Geometry: final body of the model. Coordinates: model frame, mm. A direction names the side the tool comes from. Give positions to 0.01 mm unless a question says otherwise; leave off trailing zeros. Order: outer loops, then holes, each group sorted by start corner. A loop starts at its lowest first (then second) coordinate and runs counter-clockwise, first axis right, second up. Notation, with made-up numbers: (20, 83.5) - (79, 83.5) arc R29 ccw to (79, 106.5) - close; hole circle Ø6 at (87.25, 8.25). An arc over 180 degrees is marked (long way). One line per item, written item: value.
```python
from build123d import *

# Parameters (mm, degrees)
PAD_DEPTH    = 5
CHAMFER_SIZE = 1


with BuildPart() as part:
    # Sketch → Pad (new body)
    with BuildSketch(Plane.XY):
        with BuildLine():
            Line((-27.004105, 1.5), (27.004105, 1.5))
            ThreePointArc((27.004105, 1.5), (31.989773, 6.514332), (26.975441, 11.5))
            Line((26.975441, 11.5), (10.000461, 11.451343))
            Line((10.000461, 11.451343), (10.000461, 14.500006))
            Line((10.000461, 14.500006), (27.000461, 14.500006))
            ThreePointArc((27.004105, -1.5), (34.989786, 6.501822), (27.000461, 14.500006))
            Line((-27.016258, -1.5), (27.004105, -1.5))
            ThreePointArc((-27.016258, -1.5), (-36.936523, -11.509751), (-26.996758, -21.500137))
            Line((-26.996758, -21.500137), (-14.868309, -21.500137))
            Line((-14.868309, -21.500137), (-14.868309, -24.5))
            Line((-14.868309, -24.5), (-26.868309, -24.5))
            ThreePointArc((-27.004105, 1.5), (-40.004282, -11.568254), (-26.868309, -24.5))
        make_face()
    extrude(amount=PAD_DEPTH)

    # Chamfer
    chamfer_edges = [part.edges().sort_by_distance(p)[0] for p in [
        (-14.868309, -21.500137, 2.5),
        (-14.868309, -24.5, 2.5),
        (10.000461, 11.451343, 2.5),
        (10.000461, 14.500006, 2.5),
    ]]
    chamfer(chamfer_edges, length=CHAMFER_SIZE)


solid = part.part
```
1) First-contact query: pin 1 (2.5 mm diameter, centred on x = -5.5, z = 2, fed in from -Y); pin 2 (2 mm diameter, centred on y = -3.5, z = 1.5, fed in from +X); pin 3 (0.5 mm diameter, centred on y = -23, z = 3.5, fed in from +X). Flat tips, straight axial feed; report the tip coordinate or a pass-through.
Answers below:
pin 1: y = -1.5
pin 2: x = -31.3
pin 3: x = -14.87
2) Section A-A, the plane x = -18.5. Return loops of the section in (y, z), then the cut area to 3 significant figures.
Answers below:
outline: (-24.5, 0) - (-21.5, 0) - (-21.5, 5) - (-24.5, 5) - close; (-1.5, 0) - (1.5, 0) - (1.5, 5) - (-1.5, 5) - close
area: 30.0 mm^2
3) Section D-D, the plane x = 29.5. Return loops of the section in (y, z).
Answers below:
outline: (-1.1, 0) - (2.18, 0) - (2.18, 5) - (-1.1, 5) - close; (10.82, 0) - (14.1, 0) - (14.1, 5) - (10.82, 5) - close
4) Section B-B, the plane z = 4.15. Return loops of the section in (x, y).
Answers below:
outline: (-27.02, -1.5) - (27, -1.5) arc R8 ccw to (27, 14.5) - (11, 14.5) - (10, 13.5) - (10, 12.45) - (11, 11.45) - (26.98, 11.5) arc R5 cw to (27, 1.5) - (-27, 1.5) arc R13 ccw (long way) to (-26.87, -24.5) - (-15.87, -24.5) - (-14.87, -23.5) - (-14.87, -22.5) - (-15.87, -21.5) - (-27, -21.5) arc R10 cw to start
5) Mould query, pull axis Y, two halves, no side actions, for faces 4 (the face through (34.988, 6.326, 2.465)), 5 (the face through (-36.934, -11.291, 2.465)), 6 (the face through (-2, -1, 0)). Classes: released by +Y, released by -Y, zero draft, split by the parting line, or undercut.
Answers below:
face 4: split by the parting line
face 5: undercut
face 6: zero draft
6) Material intervals for line 1 along Y through (x, z) = (-21, 2.35); line 2 along Y through (x, z) = (12, 0.2); line 3 along Y through (x, z) = (-8.5, 3.5), sorted ascending.
Answers below:
line 1: -24.5 to -21.5, -1.5 to 1.5
line 2: -1.5 to 1.5, 11.46 to 14.5
line 3: -1.5 to 1.5
7) Section C-C, the plane y = 6.5. Return loops of the section in (x, z).
Answers below:
outline: (31.99, 0) - (34.99, 0) - (34.99, 5) - (31.99, 5) - close
8) Set-up query: faces 1 (the face through (-22, -21.5, 2)), 2 (the face through (-2, -1, 5)), 3 (the face through (0, 1.5, 2)). Return all of +Z, -Z, +X, -X, +Y, -Y with unobstructed straight access to the full face (end or side cutting, diameter ignored); none if empty.
Answers below:
face 1: +Z, -Z, +X
face 2: +Z, +X, -X, +Y, -Y
face 3: +Z, -Z, -X
